from build123d import *

# Parameters (mm, degrees)
SKETCH_1_W          = 88
SKETCH_1_H          = 30
EXTRUDE_1_DEPTH     = 32.5
SKETCH_2_R          = 1.5
CUT_EXTRUDE_1_DEPTH = 57.72080747
SKETCH_3_W          = 60
SKETCH_3_H          = 30
CUT_EXTRUDE_2_DEPTH = 25


with BuildPart() as part:
    # 草图1 → 凸台-拉伸1 (new body)
    with BuildSketch(Plane(origin=(0, 0, 0), x_dir=(1, 0, 0), z_dir=(0, 1, 0))):
        Rectangle(SKETCH_1_W, SKETCH_1_H)
    extrude(amount=EXTRUDE_1_DEPTH)

    # 草图2 → 切除-拉伸1 (cut, through all)
    with BuildSketch(Plane(origin=(0, 32.5, 0), x_dir=(1, 0, 0), z_dir=(0, 1, 0))):
        with Locations(Location((-25, 0, 0), (0, 0, 270))):
            Circle(SKETCH_2_R)
        with Locations(Location((25, 0, 0), (0, 0, 90))):
            Circle(SKETCH_2_R)
    extrude(amount=-CUT_EXTRUDE_1_DEPTH, mode=Mode.SUBTRACT)

    # 草图3 → 切除-拉伸2 (cut)
    with BuildSketch(Plane(origin=(0, 32.5, 0), x_dir=(1, 0, 0), z_dir=(0, 1, 0))):
        Rectangle(SKETCH_3_W, SKETCH_3_H)
    extrude(amount=-CUT_EXTRUDE_2_DEPTH, mode=Mode.SUBTRACT)


solid = part.part
Build history of the part. All positions in model axes, mm. A direction names the side the tool comes from. Coordinates: 2 decimals unless noted, no trailing zeros. Write each loop counter-clockwise with the first axis right and the second up, starting at its lowest first coordinate (ties: lowest second). Pieces come first, ordered by that corner, then holes.
(1) Drill centre lines: line 1 (X direction, y = 3, z = 0); line 2 (Z direction, x = 25, y = 3); line 3 (X direction, y = 22, z = 9.5). Where is each one in solid material? Low to high.
(2) 3-axis set-ups, long thin cutter, end or side, ignore diameter. For faces 4 (the flat face through (37, 32.5, 0)), 5 (the flat face through (0, 7.5, 0)): which of +Z, -Z, +X, -X, +Y, -Y reach the whole face in a straight line?
(3) Cut at A-A on y = 20.5. List the corners of the cut face in (x, z).
(4) Cut at C-C on x = 25. List the corners of the cut face in (y, z), and give its area (4 significant figures).
(5) Mould opens along Z. For faces 1 (the flat face through (30, 20, 0)), 2 (the flat face through (-1, 5, -15)), 3 (the cylindrical face through (-23.513, 3.803, -0.195)) say: pulls with the +Z half, pulls with the -Z half, needs draft (parallel to the pull), parting line crosses it, or undercut.
(6) Pin check, flat tip, straight feed: pin 1 Ø3.5 at (x, z) = (-25, 0) entering from +Y. Stop position of the tip, or through.
(7) Cut at D-D on z = 7.5. List the corners of the cut face in (x, y), and give its area (3 significant figures).
(8) Cut at B-B on z = 0. List the corners of the cut face in (x, y), and give its area (4 significant figures).
Working result:
1. line 1: x = -44 to -26.5, -23.5 to 23.5, 26.5 to 44
1. line 2: z = -15 to -1.5, 1.5 to 15
1. line 3: x = -44 to -30, 30 to 44
2. face 4: +Z, -Z, +X, -X, +Y
2. face 5: +Z, -Z, +Y
3. outline: (-44, -15) - (-30, -15) - (-30, 15) - (-44, 15) - close; (30, -15) - (44, -15) - (44, 15) - (30, 15) - close
4. outline: (0, -15) - (7.5, -15) - (7.5, -1.5) - (0, -1.5) - close; (0, 1.5) - (7.5, 1.5) - (7.5, 15) - (0, 15) - close
4. area: 202.5 mm2
5. face 1: needs draft
5. face 2: pulls with the -Z half
5. face 3: undercut
6. pin 1: stops at y = 7.5
7. outline: (-44, 0) - (44, 0) - (44, 32.5) - (30, 32.5) - (30, 7.5) - (-30, 7.5) - (-30, 32.5) - (-44, 32.5) - close
7. area: 1,360 mm2
8. outline: (-44, 0) - (-26.5, 0) - (-26.5, 7.5) - (-30, 7.5) - (-30, 32.5) - (-44, 32.5) - close; (-23.5, 0) - (23.5, 0) - (23.5, 7.5) - (-23.5, 7.5) - close; (26.5, 0) - (44, 0) - (44, 32.5) - (30, 32.5) - (30, 7.5) - (26.5, 7.5) - close
8. area: 1,315 mm2
